```python
from build123d import *

# Parameters (mm, degrees)
SKETCH1_R           = 3
BOSS_EXTRUDE1_DEPTH = 16


with BuildPart() as part:
    # Sketch1 → Boss-Extrude1 (new, symmetric)
    with BuildSketch(Plane.XY):
        with BuildLine():
            Line((-0.893039494, 6.816751826), (-5.456960506, 4.181770802))
            ThreePointArc((-5.456960506, 4.181770802), (-5.953924651, 3.4375), (-6.35, 2.634981025))
            Line((-6.35, 2.634981025), (-6.35, -2.634981025))
            ThreePointArc((-6.35, -2.634981025), (-5.953924651, -3.4375), (-5.456960506, -4.181770802))
            Line((-5.456960506, -4.181770802), (-0.893039494, -6.816751826))
            ThreePointArc((-0.893039494, -6.816751826), (0, -6.875), (0.893039494, -6.816751826))
            Line((0.893039494, -6.816751826), (5.456960506, -4.181770802))
            ThreePointArc((5.456960506, -4.181770802), (5.953924651, -3.4375), (6.35, -2.634981025))
            Line((6.35, -2.634981025), (6.35, 2.634981025))
            ThreePointArc((6.35, 2.634981025), (5.953924651, 3.4375), (5.456960506, 4.181770802))
            Line((5.456960506, 4.181770802), (0.893039494, 6.816751826))
            ThreePointArc((0.893039494, 6.816751826), (0, 6.875), (-0.893039494, 6.816751826))
        make_face()
        Circle(SKETCH1_R, mode=Mode.SUBTRACT)
    extrude(amount=BOSS_EXTRUDE1_DEPTH, both=True)


solid = part.part
```
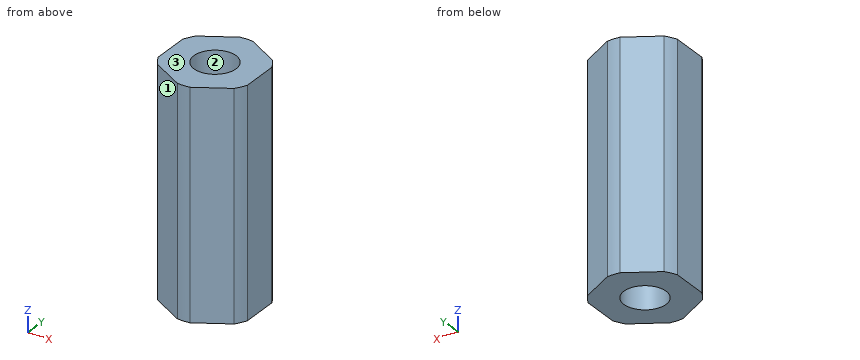
The model under review builds one solid part; all positions refer to its coordinate system, in mm. Face numbers are marked on the shaded views. Round coordinates to 2 decimals unless told otherwise and drop trailing zeros. Loops run counter-clockwise (first coordinate to the right, second up) from the corner with the lowest first, then second, coordinate; pieces in that order, holes last. Notation, with made-up numbers: M 26.25,26.25 L 51.25,26.25 A22 ccw 51.25,60.25 Z; hole C 56.25,-28.75 d6. An arc over 180 degrees is marked long. Put each result on its own line as item: value.
Q1. Consider section B-B, the plane y = 0. Give the boundary of the cut face in (x, z), then the cut area to 3 significant figures.
Result set:
outline: M -6.35,-16 L -3,-16 L -3,16 L -6.35,16 Z; M 3,-16 L 6.35,-16 L 6.35,16 L 3,16 Z
area: 214 mm²
Q2. Consider section C-C, the plane z = -3. Give the boundary of the cut face in (x, y) (3 decimals), then the cut area to 3 significant figures.
Result set:
outline: M -6.35,-2.635 A6.875 ccw -5.457,-4.182 L -0.893,-6.817 A6.875 ccw 0.893,-6.817 L 5.457,-4.182 A6.875 ccw 6.35,-2.635 L 6.35,2.635 A6.875 ccw 5.457,4.182 L 0.893,6.817 A6.875 ccw -0.893,6.817 L -5.457,4.182 A6.875 ccw -6.35,2.635 Z; hole C 0,0 d6
area: 109 mm²
Q3. Consider section A-A, the plane x = 0. Give the boundary of the cut face in (y, z) (3 decimals), then the cut area to 3 significant figures.
Result set:
outline: M -6.875,-16 L -3,-16 L -3,16 L -6.875,16 Z; M 3,-16 L 6.875,-16 L 6.875,16 L 3,16 Z
area: 248 mm²
Q4. Consider section D-D, the plane y = -5.5. Give the boundary of the cut face in (x, z).
Result set:
outline: M -3.17,-16 L 3.17,-16 L 3.17,16 L -3.17,16 Z
Q5. For pin 1 (4 mm diameter, centred on x = -3, z = -6.5, fed in from -Y) (3 decimals); pin 2 (1.5 mm diameter, centred on y = -4, z = -5, fed in from +X); pin 3 (6 mm diameter, centred on x = -3.5, z = -9.5, fed in from +Y), all flat-tipped, find the tip position at first contact; note any pin that passes through.
Result set:
pin 1: stops at y = -6.755
pin 2: stops at x = 6.06
pin 3: stops at y = 6.86
Q6. To check wall thickness, follow L1, parallel to Y at x = 0, z = 4.5 (3 decimals); L2, parallel to X at y = 1.5, z = 10; L3, parallel to Y at x = -4.5, z = -5. State the ranges of each line that lie inside material, in increasing order.
Result set:
L1: y = -6.875 to -3, 3 to 6.875
L2: x = -6.35 to -2.6, 2.6 to 6.35
L3: y = -4.73 to 4.73
Q7. Mouldability with a two-part tool opening along Y and no side actions: class the marked faces 1, 2 and 3 as released by +Y, released by -Y, zero draft, split by the parting line, or undercut.
Result set:
face 1: released by -Y
face 2: undercut
face 3: zero draft
